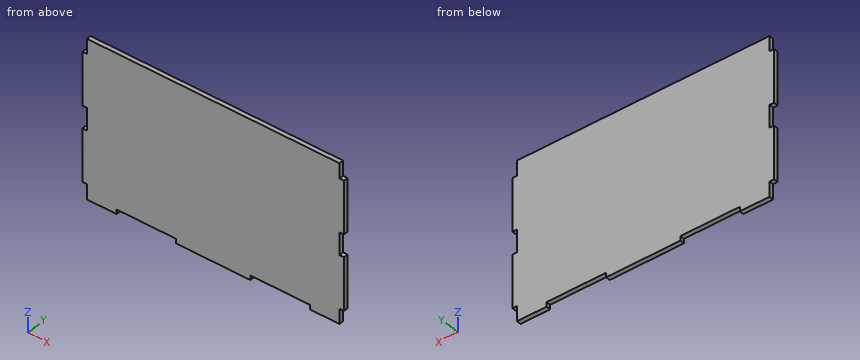
```python
from build123d import *

# Parameters (mm, degrees)
F0_W     = 3
F0_H     = 35
F1_DEPTH = 3


with BuildPart() as f1:
    # F0 (on Front) → F1 (new body)
    with BuildSketch(Plane.XZ):
        Polygon((85, 42.5), (85, 52.5), (-85, 52.5), (-85, 42.5), (-85, 7.5), (-85, -7.5), (-85, -42.5), (-85, -52.5), (-65, -52.5), (-65, -49.5), (-25, -49.5), (-25, -52.5), (25, -52.5), (25, -49.5), (65, -49.5), (65, -52.5), (85, -52.5), (85, -42.5), (85, -7.5), (85, 7.5), align=None)
        with Locations((-86.5, -25)):
            Rectangle(F0_W, F0_H)
        with Locations((86.5, -25)):
            Rectangle(F0_W, F0_H)
        with Locations((86.5, 25)):
            Rectangle(F0_W, F0_H)
        with Locations((-86.5, 25)):
            Rectangle(F0_W, F0_H)
    extrude(amount=F1_DEPTH)


solid = f1.part
```
CAD build for the part. Positions are in the model's coordinates, mm. Coordinates: 2 decimals unless noted, no trailing zeros. Write each loop counter-clockwise with the first axis right and the second up, starting at its lowest first coordinate (ties: lowest second). Pieces come first, ordered by that corner, then holes. Notation, with made-up numbers: (50.5, 87) -> (62.5, 87) arc R19 cw to (62.5, 95) -> close; hole circle Ø8 at (-14.5, -36.5). An arc over 180 degrees is marked (long way). Use CSV: the item, a comma, the result in double quotes. Start each with the question number.
Item 1: Drop flat-ended pins along their axis: P1, Ø1.5, axis at y = -1.5, z = 49.5, coming from the +X side; P2, Ø0.9, axis at x = -87, y = -2, coming from the +Z side; P3, Ø1.5, axis at x = -40.5, y = -1.5, coming from the -Z side; P4, Ø6, axis at x = 25.5, z = -11, coming from the +Y side. Give the stop position or say it passes through.
Item 2: Wall check: probe 1 along X at (y, z) = (-2.4, -1); probe 2 along Z at (x, y) = (-60, -1.4). Give the ranges that are in metal, low to high.
Item 3: Band-saw the part on A-A, the plane y = -2.05. Write the cut outline in (x, z), plus the area to 3 significant figures.
Item 4: Band-saw the part on C-C, the plane x = 53.5. Write the cut outline in (y, z).
Item 5: Band-saw the part on B-B, the plane z = 0. Write the cut outline in (x, y).
Response values:
1,P1,"stops at x = 85"
1,P2,"stops at z = 42.5"
1,P3,"stops at z = -49.5"
1,P4,"stops at y = 0"
2,probe 1,"x = -85 to 85"
2,probe 2,"z = -49.5 to 52.5"
3,outline,"(-88, -42.5) -> (-85, -42.5) -> (-85, -52.5) -> (-65, -52.5) -> (-65, -49.5) -> (-25, -49.5) -> (-25, -52.5) -> (25, -52.5) -> (25, -49.5) -> (65, -49.5) -> (65, -52.5) -> (85, -52.5) -> (85, -42.5) -> (88, -42.5) -> (88, -7.5) -> (85, -7.5) -> (85, 7.5) -> (88, 7.5) -> (88, 42.5) -> (85, 42.5) -> (85, 52.5) -> (-85, 52.5) -> (-85, 42.5) -> (-88, 42.5) -> (-88, 7.5) -> (-85, 7.5) -> (-85, -7.5) -> (-88, -7.5) -> close"
3,area,"18,000 mm2"
4,outline,"(-3, -49.5) -> (0, -49.5) -> (0, 52.5) -> (-3, 52.5) -> close"
5,outline,"(-85, -3) -> (85, -3) -> (85, 0) -> (-85, 0) -> close"
